Could you check a few things on this drawing? It's one solid part, dimensions in mm from its lowest x, y, z. A direction names the side the tool comes from. Give positions to 0.01 mm unless a question says otherwise; leave off trailing zeros. Loops run counter-clockwise (first coordinate to the right, second up) from the corner with the lowest first, then second, coordinate; pieces in that order, holes last. Notation, with made-up numbers: (33, 53) - (87, 53) arc R25 ccw to (87, 72) - close; hole circle Ø8 at (80.5, 79). An arc over 180 degrees is marked (long way). Use CSV: the item, a comma, the result in double quotes.
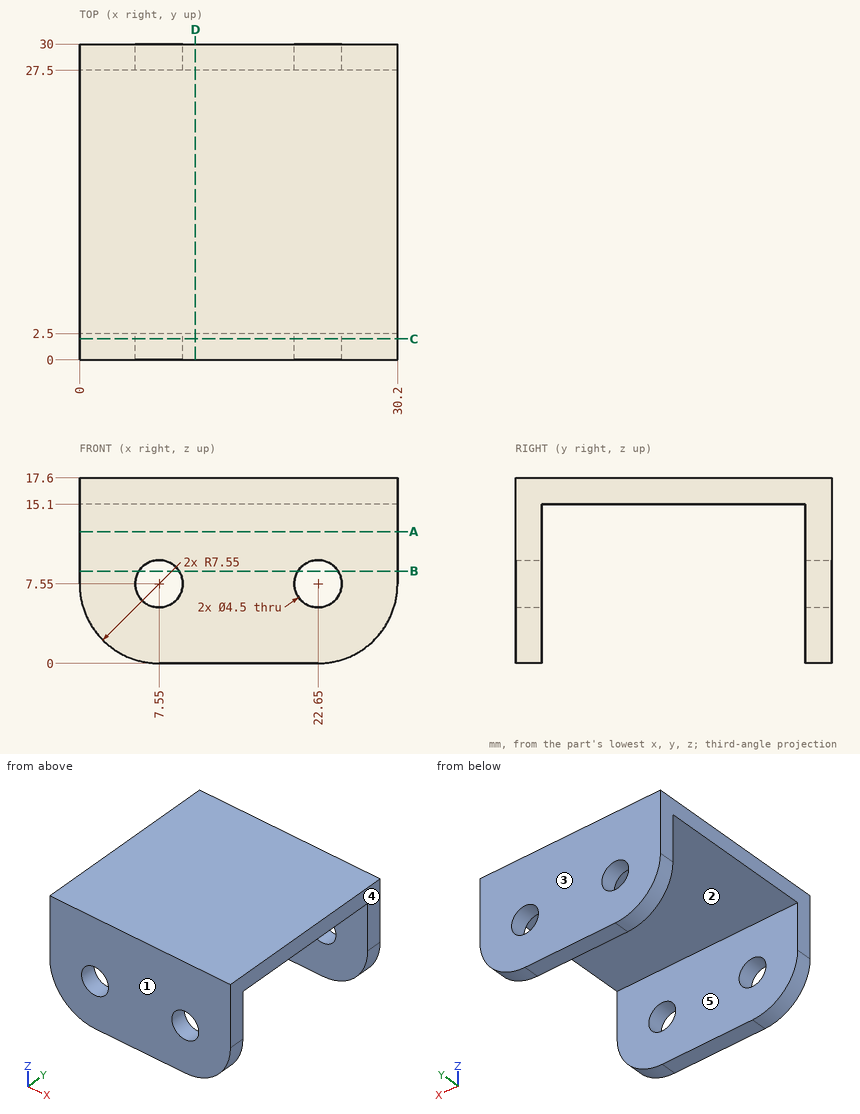
1) Suppose I cut it at A-A (z = 12.5). Please give me the cut outline in (x, y).
Answer below:
outline,"(0, 0) - (30.2, 0) - (30.2, 2.5) - (0, 2.5) - close; (0, 27.5) - (30.2, 27.5) - (30.2, 30) - (0, 30) - close"
2) I need wall thicknesses on line 1 along X through (y, z) = (0.65, 7.55); line 2 along Y through (x, z) = (26.5, 12.25); line 3 along Z through (x, y) = (22.65, 1.65). Which ranges of each line are inside material? Lowest first, please.
Answer below:
line 1,"x = 0 to 5.3, 9.8 to 20.4, 24.9 to 30.2"
line 2,"y = 0 to 2.5, 27.5 to 30"
line 3,"z = 0 to 5.3, 9.8 to 17.6"
3) I'm going to push flat-ended pins straight in: P1, Ø4, axis at x = 7.5, y = 23, coming from the -Z side; P2, Ø3.5, axis at x = 22.65, z = 7.55, coming from the +Y side. Where does each tip first touch, or does it pass through?
Answer below:
P1,"stops at z = 15.1"
P2,"passes through"
4) We'd pull the mould along Y, two halves only. Please class the marked faces 3, 4 and 5: +Y half, -Y half, draft (parallel to the pull), parting line (faces both ways), or undercut.
Answer below:
face 3,"+Y half"
face 4,"draft"
face 5,"undercut"
5) Suppose I cut it at B-B (z = 8.75). Please give me the cut outline in (x, y).
Answer below:
outline,"(0, 0) - (5.65, 0) - (5.65, 2.5) - (0, 2.5) - close; (0, 27.5) - (5.65, 27.5) - (5.65, 30) - (0, 30) - close; (9.45, 0) - (20.75, 0) - (20.75, 2.5) - (9.45, 2.5) - close; (9.45, 27.5) - (20.75, 27.5) - (20.75, 30) - (9.45, 30) - close; (24.55, 0) - (30.2, 0) - (30.2, 2.5) - (24.55, 2.5) - close; (24.55, 27.5) - (30.2, 27.5) - (30.2, 30) - (24.55, 30) - close"
6) Suppose I cut it at C-C (y = 2). Please give me the cut outline in (x, z), plus the area to 3 significant figures.
Answer below:
outline,"(0, 7.55) arc R7.55 ccw to (7.55, 0) - (22.65, 0) arc R7.55 ccw to (30.2, 7.55) - (30.2, 17.6) - (0, 17.6) - close; hole circle Ø4.5 at (7.55, 7.55); hole circle Ø4.5 at (22.65, 7.55)"
area,"475 mm2"
7) Which directions (+Z, -Z, +X, -X, +Y, -Y) give clear straight access to the entire face, cutting with the end or side of a thin tool? Please do the marked faces 1 and 2.
Answer below:
face 1,"+Z, -Z, +X, -X, -Y"
face 2,"-Z, +X, -X"
8) Suppose I cut it at D-D (x = 11). Please give me the cut outline in (y, z).
Answer below:
outline,"(0, 0) - (2.5, 0) - (2.5, 15.1) - (27.5, 15.1) - (27.5, 0) - (30, 0) - (30, 17.6) - (0, 17.6) - close"
